The model under review builds one solid part; all positions refer to its coordinate system, in mm. A direction names the side the tool comes from. Give positions to 0.01 mm unless a question says otherwise; leave off trailing zeros. Loops run counter-clockwise (first coordinate to the right, second up) from the corner with the lowest first, then second, coordinate; pieces in that order, holes last. Notation, with made-up numbers: M 68.25,74 L 114.25,74 A23 cw 114.25,108 Z; hole C 39.5,-33 d9. An arc over 180 degrees is marked long. Write item = value, one per line. Start each with the question number.
1. We need section D-D on z = -13. Give the boundary of the cut face in (x, y).
2. Wall thickness on line 1 along Z through (x, y) = (9.25, 3.25); line 2 along X through (y, z) = (13.5, -17.5); line 3 along Z through (x, y) = (18.75, 18): over which ranges is each line inside the solid? List them lowest first. Write a range as from..to.
3. We need section A-A on x = 22.5. Give the boundary of the cut face in (y, z), then the cut area to 3 significant figures.
4. For pin 1 (6 mm diameter, centred on x = 19.5, y = 11, fed in from +Z); pin 2 (8 mm diameter, centred on x = 6.5, y = 11.5, fed in from +Z); pin 3 (10 mm diameter, centred on x = 20, y = 5, fed in from -Z); pin 4 (12 mm diameter, centred on x = 19.5, z = -10.5, fed in from -Y), all flat-tipped, find the tip position at first contact; note any pin that passes through.
5. We need section C-C on y = 4.5. Give the boundary of the cut face in (x, z).
6. For faces 1 (the face through (0, 10, -10)), 2 (the face through (6.358, 2.433, 3.698)), 3 (the face through (17.4, 1.55, -8.97)), list the 3-axis set-ups (+Z, -Z, +X, -X, +Y, -Y) from which the entire face can be reached by the end or side of a thin tool; tool diameter is ignored.
7. Draft analysis for pull direction Y (two halves, no side actions). For faces 4 (the face through (5, 10, 0)), 5 (the face through (25, 18, -10)), 6 (the face through (5, 20, -10)), state which applies: pulls with the +Y half, pulls with the -Y half, needs draft (parallel to the pull), parting line crosses it, or undercut.
8. We need section B-B on z = 0.5. Give the boundary of the cut face in (x, y).
from build123d import *

# Parameters (mm, degrees)
SKETCH2_W           = 10
SKETCH2_H           = 20
BOSS_EXTRUDE1_DEPTH = 20
SKETCH3_R           = 1.5
BOSS_EXTRUDE2_DEPTH = 7.5
SKETCH6_R           = 1.5
BOSS_EXTRUDE4_DEPTH = 15
SKETCH8_R           = 1.5
BOSS_EXTRUDE5_DEPTH = 15


with BuildPart() as part:
    # Sketch2 → Boss-Extrude1 (new body)
    with BuildSketch(Plane(origin=(0, 0, 0), x_dir=(1, 0, 0), z_dir=(0, 1, 0))):
        with Locations((5, 10)):
            Rectangle(SKETCH2_W, SKETCH2_H)
    extrude(amount=BOSS_EXTRUDE1_DEPTH)

    # Sketch3 → Boss-Extrude2 (add)
    with BuildSketch(Plane.XY):
        with Locations(Location((5.252029318, 3.447237738, 0), (0, 0, 180))):
            Circle(SKETCH3_R)
        with Locations(Location((5.252029318, 17.447237738, 0), (0, 0, 180))):
            Circle(SKETCH3_R)
    extrude(amount=BOSS_EXTRUDE2_DEPTH)

    # Sketch6 → Boss-Extrude4 (add)
    with BuildSketch(Plane(origin=(10, 0, 0), x_dir=(0, 0, -1), z_dir=(1, 0, 0))):
        with Locations(Location((10.400607827, 2, 0), (0, 0, 180))):
            Circle(SKETCH6_R)
    extrude(amount=BOSS_EXTRUDE4_DEPTH)

    # Sketch8 → Boss-Extrude5 (add)
    with BuildSketch(Plane(origin=(10, 0, 0), x_dir=(0, 0, -1), z_dir=(1, 0, 0))):
        with Locations(Location((10.400607827, 18, 0), (0, 0, 180))):
            Circle(SKETCH8_R)
    extrude(amount=BOSS_EXTRUDE5_DEPTH)


solid = part.part
Final values:
q1.outline = M 0,0 L 10,0 L 10,20 L 0,20 Z
q2.line_1 = -20..0
q2.line_2 = 0..10
q2.line_3 = -11.9..-8.9
q3.outline = C 2,-10.4 d3; C 18,-10.4 d3
q3.area = 14.1 mm²
q4.pin_1 = through
q4.pin_2 = 0
q4.pin_3 = -11.9
q4.pin_4 = 0.5
q5.outline = M 0,-20 L 10,-20 L 10,0 L 6.32,0 L 6.32,7.5 L 4.18,7.5 L 4.18,0 L 0,0 Z
q6.face_1 = +Z, -Z, -X, +Y, -Y
q6.face_2 = +Z
q6.face_3 = +X
q7.face_4 = undercut
q7.face_5 = needs draft
q7.face_6 = pulls with the +Y half
q8.outline = C 5.25,3.45 d3; C 5.25,17.45 d3
